from build123d import *

# Parameters (mm, degrees)
BOSS_EXTRUDE1_DEPTH = 7.5
SKETCH2_W           = 150
SKETCH2_H           = 2.5
BOSS_EXTRUDE2_DEPTH = 20
SKETCH3_R           = 1.4
CUT_EXTRUDE1_DEPTH  = 10
SKETCH4_R           = 3
BOSS_EXTRUDE3_DEPTH = 20
SKETCH5_R           = 1.4
CUT_EXTRUDE2_DEPTH  = 8


with BuildPart() as part:
    # Sketch1 → Boss-Extrude1 (new body)
    with BuildSketch(Plane(origin=(0, 0, 0), x_dir=(1, 0, 0), z_dir=(0, 1, 0))):
        with BuildLine():
            Line((-150, 85), (-25, 85))
            ThreePointArc((-25, 85), (-17.67766953, 67.32233047), (0, 60))
            Line((0, 60), (0, 0))
            Line((0, 0), (-150, 0))
            Line((-150, 0), (-150, 85))
        make_face()
    extrude(amount=BOSS_EXTRUDE1_DEPTH)

    # Sketch2 → Boss-Extrude2 (add)
    with BuildSketch(Plane(origin=(0, 7.5, 0), x_dir=(1, 0, 0), z_dir=(0, 1, 0))):
        with Locations((-75, 23.75)):
            Rectangle(SKETCH2_W, SKETCH2_H)
        with Locations((-75, 28.95)):
            Rectangle(SKETCH2_W, SKETCH2_H)
    extrude(amount=BOSS_EXTRUDE2_DEPTH)

    # Sketch3 → Cut-Extrude1 (cut)
    with BuildSketch(Plane.XY.offset(-22.5)):
        with Locations((-30, 25)):
            Circle(SKETCH3_R)
        with Locations((-5, 25)):
            Circle(SKETCH3_R)
        with Locations((-30, 15)):
            Circle(SKETCH3_R)
        with Locations((-5, 15)):
            Circle(SKETCH3_R)
        with Locations((-145, 15)):
            Circle(SKETCH3_R)
        with Locations((-120, 15)):
            Circle(SKETCH3_R)
        with Locations((-145, 25)):
            Circle(SKETCH3_R)
        with Locations((-120, 25)):
            Circle(SKETCH3_R)
    extrude(amount=-CUT_EXTRUDE1_DEPTH, mode=Mode.SUBTRACT)

    # Sketch4 → Boss-Extrude3 (add)
    with BuildSketch(Plane(origin=(0, 7.5, 0), x_dir=(1, 0, 0), z_dir=(0, 1, 0))):
        with Locations(Location((-78, 42.75, 0), (0, 0, 270))):
            Circle(SKETCH4_R)
        with Locations(Location((-20, 42.75, 0), (0, 0, 270))):
            Circle(SKETCH4_R)
        with Locations(Location((-135, 7.75, 0), (0, 0, 270))):
            Circle(SKETCH4_R)
    extrude(amount=BOSS_EXTRUDE3_DEPTH)

    # Sketch5 → Cut-Extrude2 (cut)
    with BuildSketch(Plane(origin=(0, 27.5, 0), x_dir=(1, 0, 0), z_dir=(0, 1, 0))):
        with Locations(Location((-78, 42.75, 0), (0, 0, 270))):
            Circle(SKETCH5_R)
        with Locations(Location((-20, 42.75, 0), (0, 0, 270))):
            Circle(SKETCH5_R)
        with Locations(Location((-135, 7.75, 0), (0, 0, 270))):
            Circle(SKETCH5_R)
    extrude(amount=-CUT_EXTRUDE2_DEPTH, mode=Mode.SUBTRACT)


solid = part.part
The listing builds one solid part. Answer for the finished solid, in the listing's coordinates (mm). A direction names the side the tool comes from. Coordinates: 2 decimals unless noted, no trailing zeros. Order: outer loops, then holes, each group sorted by start corner. A loop starts at its lowest first (then second) coordinate and runs counter-clockwise, first axis right, second up. Notation, with made-up numbers: (-19.75, 64) -> (18.25, 64) arc R13 ccw to (18.25, 85) -> close; hole circle Ø3 at (-22.75, 9). An arc over 180 degrees is marked (long way). Answer in a Markdown table with one row per item. Add a question column.
Item 1: Find section A-A (x = -145). Write down the section's boundary in (y, z), then the cut area to 4 significant figures.
Item 2: Find section B-B (y = 25). State how many separate pieces and enclosed holes the cut face has, then the cut area to 3 significant figures.
Item 3: Determine the mould class of faces 3 (the face through (-88, 4, -85)), 4 (the face through (-76, 17, -25)), 5 (the face through (-146.4, 25.06, -23.73)) for opening direction Z: +Z half, -Z half, draft (parallel to the pull), parting line (faces both ways), or undercut.
Item 4: Find section C-C (x = -58.5). Write down the section's boundary in (y, z), then the cut area to 4 significant figures.
Item 5: Which of the six approach directions +Z, -Z, +X, -X, +Y, -Y give full straight-line access (tool end or side, diameter ignored) to faces 1 (the face through (-132.47, 17.36, -6.14)), 2 (the face through (-136, 27.5, -6))?
Item 6: Find section D-D (z = -42.75). Write down the section's boundary in (x, y).
Item 7: Each of these flat-tipped pins is pushed along its axis until it touches: P1, Ø3, axis at x = -30, y = 15, coming from the +Z side; P2, Ø2, axis at x = -101, z = -17, coming from the +Y side; P3, Ø2.5, axis at x = -5, y = 15, coming from the +Z side; P4, Ø3, axis at x = -30, y = 25, coming from the -Z side. Where does it stop, or does it pass through?
Item 8: Find the intervals of material crossed by L1, parallel to Y at x = -30, z = -29.6; L2, parallel to X at y = 25.25, z = -42.75; L3, parallel to Z at x = -29, y = 11.5, in increasing order. Write a range as from..to.
Result set:
| question | item | result |
|---|---|---|
| 1 | outline | (0, -85) -> (7.5, -85) -> (7.5, -30.2) -> (13.6, -30.2) -> (13.6, -27.7) -> (7.5, -27.7) -> (7.5, -25) -> (13.6, -25) -> (13.6, -22.5) -> (7.5, -22.5) -> (7.5, 0) -> (0, 0) -> close; (16.4, -30.2) -> (23.6, -30.2) -> (23.6, -27.7) -> (16.4, -27.7) -> close; (16.4, -25) -> (23.6, -25) -> (23.6, -22.5) -> (16.4, -22.5) -> close; (26.4, -30.2) -> (27.5, -30.2) -> (27.5, -27.7) -> (26.4, -27.7) -> close; (26.4, -25) -> (27.5, -25) -> (27.5, -22.5) -> (26.4, -22.5) -> close |
| 1 | area | 709.5 mm² |
| 2 | separate pieces | 13 |
| 2 | enclosed holes | 3 |
| 2 | area | 760 mm² |
| 3 | face 3 | -Z half |
| 3 | face 4 | undercut |
| 3 | face 5 | draft |
| 4 | outline | (0, -85) -> (7.5, -85) -> (7.5, -30.2) -> (27.5, -30.2) -> (27.5, -27.7) -> (7.5, -27.7) -> (7.5, -25) -> (27.5, -25) -> (27.5, -22.5) -> (7.5, -22.5) -> (7.5, 0) -> (0, 0) -> close |
| 4 | area | 737.5 mm² |
| 5 | face 1 | +Y |
| 5 | face 2 | +Z, -Z, +X, -X, +Y |
| 6 | outline | (-150, 0) -> (0, 0) -> (0, 7.5) -> (-17, 7.5) -> (-17, 27.5) -> (-18.6, 27.5) -> (-18.6, 19.5) -> (-21.4, 19.5) -> (-21.4, 27.5) -> (-23, 27.5) -> (-23, 7.5) -> (-75, 7.5) -> (-75, 27.5) -> (-76.6, 27.5) -> (-76.6, 19.5) -> (-79.4, 19.5) -> (-79.4, 27.5) -> (-81, 27.5) -> (-81, 7.5) -> (-150, 7.5) -> close |
| 7 | P1 | stops at z = -22.5 |
| 7 | P2 | stops at y = 7.5 |
| 7 | P3 | passes through |
| 7 | P4 | stops at z = -30.2 |
| 8 | L1 | y = 0..13.6, 16.4..23.6, 26.4..27.5 |
| 8 | L2 | x = -81..-79.4, -76.6..-75, -23..-21.4, -18.6..-17 |
| 8 | L3 | z = -30.2..-27.7, -25..-22.5 |
